from build123d import *

# Parameters (mm, degrees)
F0_R     = 5
F1_ANGLE = 45
F2_R     = 17.5
F2_R_2   = 5
F3_DEPTH = 1
F5_ANGLE = 135
F7_ANGLE = 45


with BuildPart() as f1:
    # F0 (on Top) → F1 (revolve)
    with BuildSketch(Plane.XY):
        with Locations((17.2625295818, 39.9485491216)):
            Circle(F0_R)
    revolve(axis=Axis((11.3439466804, 38.7977138162, 0), (0, -1, 0)), revolution_arc=F1_ANGLE)

    # F2 (on face) → F3 (join)
    with BuildSketch(Plane(origin=(0, 0, 0), x_dir=(1, 0, 0), z_dir=(0, 0, -1))):
        with Locations((17.2625295818, -39.9485491216)):
            Circle(F2_R)
        with Locations((17.2625295818, -39.9485491216)):
            Circle(F2_R_2, mode=Mode.SUBTRACT)
        with Locations((17.2625295818, -39.9485491216)):
            Circle(F2_R_2)
    extrude(amount=F3_DEPTH)

    # F4 (on face) → F5 (revolve)
    with BuildSketch(Plane(origin=(0, 0, -1), x_dir=(1, 0, 0), z_dir=(0, 0, -1))):
        Polygon((12.9011229654, -29.9485491216), (2.9011229654, -29.9485491216), (2.9011229654, -49.9485491216), (12.9011229654, -49.9485491216), (12.9011229654, -44.1824280606), (21.6239361981, -44.1824280606), (21.6239361981, -49.9485491216), (31.6239361981, -49.9485491216), (31.6239361981, -29.9485491216), (21.6239361981, -29.9485491216), (21.6239361981, -36.1191299331), (12.9011229654, -36.1218505295), align=None)
    revolve(axis=Axis((-26.9732894376, 40.484293364, -1), (0, 1, 0)), revolution_arc=F5_ANGLE)

    # F6 (on face) → F7 (revolve)
    with BuildSketch(Plane(origin=(-12.9866447188, 0, 12.9866447188), x_dir=(0, -1, 0), z_dir=(-0.7071067812, 0, 0.7071067812))):
        Polygon((-36.1218505295, -59.6545150564), (-29.9485491216, -59.6545150564), (-29.9485491216, -49.6545150564), (-49.9485491216, -49.6545150564), (-49.9485491216, -59.6545150564), (-44.1824280606, -59.6545150564), (-44.1824280606, -68.3773282891), (-49.9485491216, -68.3773282891), (-49.9485491216, -78.3773282891), (-29.9485491216, -78.3773282891), (-29.9485491216, -68.3773282891), (-36.1191299331, -68.3773282891), align=None)
    revolve(axis=Axis((-81.8073011532, 42.3686988652, -55.8340117156), (0, -1, 0)), revolution_arc=F7_ANGLE)


solid = f1.part
Design review of the part built by this model. Coordinates are the model's own, in mm. A direction names the side the tool comes from. Coordinates: 2 decimals unless noted, no trailing zeros. Write each loop counter-clockwise with the first axis right and the second up, starting at its lowest first coordinate (ties: lowest second). Pieces come first, ordered by that corner, then holes. Notation, with made-up numbers: (-17.75, 21) - (37.25, 21) arc R19 ccw to (37.25, 42) - close; hole circle Ø7 at (66.25, -20). An arc over 180 degrees is marked (long way). Use one line per item in the form item = value.
Q1. For probe 1 along X at (y, z) = (44.5, -42); probe 2 along Y at (x, z) = (24, -3); probe 3 along X at (y, z) = (39, -28), list the stretches that pass through material, from the lowest coordinate up.
Taken from the geometry:
probe_1 = -68.86 to -53.06, -0.88 to 14.89
probe_2 = 29.95 to 49.95
probe_3 = -81.81 to -39.76, -14.19 to 25.03
Q2. Consider section C-C (y = 52). Write out the cut boundary in (x, z), plus the area to 3 significant figures.
Taken from the geometry:
outline = (4.57, -1) - (29.95, -1) - (29.95, 0) - (4.57, 0) - close
area = 25.4 mm^2
Q3. The part is to be moulded in two halves that separate along X. For faces 5 (the flat face through (17, 29, -1)), 6 (the flat face through (-28, 49.949, -33)), 7 (the flat face through (15.48, 40.019, 4.136)), say which applies: +X half, -X half, draft (parallel to the pull), parting line (faces both ways), or undercut.
Taken from the geometry:
face_5 = undercut
face_6 = draft
face_7 = -X half
Q4. Insertion check: pin 1 Ø3 at (x, y) = (-63, 47) entering from +Z; pin 2 Ø1 at (x, y) = (-34, 33.5) entering from +Z; pin 3 Ø6 at (x, y) = (-45, 41.5) entering from +Z. Each pin has a flat end and moves straight along its axis. Give the tip position at first contact, or say it passes through.
Taken from the geometry:
pin_1 = -11.41
pin_2 = -29.91
pin_3 = -22.22
Q5. Consider section B-B (z = -53). Write out the cut boundary in (x, y).
Taken from the geometry:
outline = (-53.99, 29.95) - (0.04, 29.95) - (0.04, 49.95) - (-53.99, 49.95) - close
Q6. Machinability: for faces 1 (the flat face through (33, 40, -1)), 2 (the flat face through (-16, 49.949, -50)), 3 (the cylindrical face through (-11.109, 47.025, -37.582)), 4 (the flat face through (-16, 29.949, -50)), which of the approach directions +Z, -Z, +X, -X, +Y, -Y give a long, thin tool a straight path to every point of the face, cutting with its end or side? Answer none if there is none.
Taken from the geometry:
face_1 = -Z, +X, +Y, -Y
face_2 = -Z, +X, -X, +Y
face_3 = +Y
face_4 = -Z, +X, -X, -Y
Q7. Consider section A-A (y = 38). Write out the cut boundary in (x, z).
Taken from the geometry:
outline = (-81.81, -36.88) arc R18.95 cw to (-68.41, -42.43) arc R58.6 ccw to (31.62, -1) - (34.65, -1) - (34.65, 0) - (21.87, 0) arc R10.52 ccw to (18.79, 7.44) - (12.27, 0.93) arc R1.31 cw to (12.66, 0) - (-0.13, 0) - (-0.13, -1) - (2.9, -1) arc R29.87 cw to (-48.1, -22.12) arc R47.67 ccw to (-81.81, -8.16) - close
